CAD build for the part. Positions are in the model's coordinates, mm. A direction names the side the tool comes from. Round coordinates to 2 decimals unless told otherwise and drop trailing zeros. Loops run counter-clockwise (first coordinate to the right, second up) from the corner with the lowest first, then second, coordinate; pieces in that order, holes last.
from build123d import *

# Parameters (mm, degrees)
SKETCH1_R           = 1.75
BOSS_EXTRUDE1_DEPTH = 15
SKETCH10_R          = 1.25
CUT_EXTRUDE3_DEPTH  = 35.960692213
SKETCH11_R          = 1.95
CUT_EXTRUDE4_DEPTH  = 47.58229165
SKETCH12_R          = 3.5
BOSS_EXTRUDE8_DEPTH = 5
BOSS_EXTRUDE9_DEPTH = 15
SKETCH14_R          = 2.75
CUT_EXTRUDE5_DEPTH  = 37.697714159
FILLET1_R           = 3
FILLET2_R           = 1.5
SKETCH15_R          = 3.5
CUT_EXTRUDE6_DEPTH  = 13


with BuildPart() as part:
    # Sketch1 → Boss-Extrude1 (new body)
    with BuildSketch(Plane(origin=(0, 0, 0), x_dir=(1, 0, 0), z_dir=(0, 1, 0))):
        with BuildLine():
            Line((-4.795571708, -25.41509434), (-11.988929271, -1.037735849))
            ThreePointArc((-11.988929271, -1.037735849), (0, 15), (11.988929271, -1.037735849))
            Line((11.988929271, -1.037735849), (4.795571708, -25.41509434))
            ThreePointArc((4.795571708, -25.41509434), (0, -29), (-4.795571708, -25.41509434))
        make_face()
        with Locations(Location((0, -24, 0), (0, 0, 270))):
            Circle(SKETCH1_R, mode=Mode.SUBTRACT)
        Polygon((0, -6.437455501), (5.575, -3.218727751), (5.575, 3.218727751), (0, 6.437455501), (-5.575, 3.218727751), (-5.575, -3.218727751), align=None, mode=Mode.SUBTRACT)
    extrude(amount=BOSS_EXTRUDE1_DEPTH)

    # Sketch10 → Cut-Extrude3 (cut, through all)
    with BuildSketch(Plane(origin=(0, 0, 0), x_dir=(1, 0, 0), z_dir=(0, 1, 0))):
        with Locations(Location((0, -13, 0), (0, 0, 270))):
            Circle(SKETCH10_R)
    extrude(amount=CUT_EXTRUDE3_DEPTH, mode=Mode.SUBTRACT)

    # Sketch11 → Cut-Extrude4 (cut, through all)
    with BuildSketch(Plane(origin=(7.806004581, 0, 24.148129883), x_dir=(0.5735764363510473, 0, 0.819152044288991), z_dir=(-0.819152044288991, 0, 0.5735764363510473))):
        with Locations((-13.609353673, 7.5)):
            Circle(SKETCH11_R)
    extrude(amount=-CUT_EXTRUDE4_DEPTH, mode=Mode.SUBTRACT)

    # Sketch12 → Boss-Extrude8 (add)
    with BuildSketch(Plane(origin=(0, 0, 0), x_dir=(1, 0, 0), z_dir=(0, 1, 0))):
        Polygon((5.575, -3.218727751), (5.575, 3.218727751), (0, 6.437455501), (-5.575, 3.218727751), (-5.575, -3.218727751), (0, -6.437455501), align=None)
        with Locations(Location((0, 0, 0), (0, 0, 270))):
            Circle(SKETCH12_R, mode=Mode.SUBTRACT)
    extrude(amount=BOSS_EXTRUDE8_DEPTH)

    # Sketch13 → Boss-Extrude9 (add)
    with BuildSketch(Plane(origin=(0, 0, 0), x_dir=(1, 0, 0), z_dir=(0, 1, 0))):
        Polygon((-19.091883092, 13.435028843), (-26.162950904, 6.363961031), (-8, -11.798989873), (-8, 2.343145751), align=None)
    extrude(amount=BOSS_EXTRUDE9_DEPTH)

    # Sketch14 → Cut-Extrude5 (cut, through all)
    with BuildSketch(Plane(origin=(-9.899494937, 0, 9.899494937), x_dir=(0.707106781186549, 0, 0.707106781186546), z_dir=(-0.707106781186546, 0, 0.707106781186549))):
        with Locations((-18, 7.5)):
            Circle(SKETCH14_R)
    extrude(amount=-CUT_EXTRUDE5_DEPTH, mode=Mode.SUBTRACT)

    # Fillet1
    # the kernel refuses this fillet: 3 mm, written as the material it takes off along each edge
    with BuildSketch(Plane(origin=(-19.091883092, -7.5, -13.435028843), x_dir=(0.7071067811865492, 0, 0.7071067811865457), z_dir=(0, 1, 0))) as fillet1_piece_1:
        with BuildLine():
            CenterArc((FILLET1_R, -FILLET1_R), FILLET1_R, 90, 90)
            Line((0, -FILLET1_R), (0, 0))
            Line((0, 0), (FILLET1_R, 0))
        make_face()
    extrude(amount=30, mode=Mode.SUBTRACT)

    # Fillet2
    fillet2_edges = [part.edges().sort_by_distance(p)[0] for p in [
        (-9.153981014, 7.5, 10.645008859),
        (-11.920074413, 7.5, -6.263220163),
    ]]
    fillet(fillet2_edges, radius=FILLET2_R)

    # Sketch15 → Cut-Extrude6 (cut)
    with BuildSketch(Plane(origin=(10.275038851, 0, -7.194659659), x_dir=(0, -1, 0), z_dir=(0.819152044288991, 0, -0.5735764363510473))):
        with Locations(Location((-7.5, -10.648976576, 0), (0, 0, 90))):
            Circle(SKETCH15_R)
    extrude(amount=-CUT_EXTRUDE6_DEPTH, mode=Mode.SUBTRACT)


solid = part.part
Item 1: Cut at A-A (y = 13). List the corners of the cut face in (x, z) (3 decimals).
Verdict:
outline: (-26.163, -6.364) - (-21.213, -11.314) arc R3 ccw to (-16.971, -11.314) - (-13.507, -7.85) arc R1.5 cw to (-11.113, -8.224) arc R12.5 ccw to (11.989, 1.038) - (4.796, 25.415) arc R5 ccw to (-4.796, 25.415) - (-9.046, 11.011) arc R1.5 cw to (-9.424, 10.375) - close; hole (-5.575, -3.219) - (0, -6.437) - (5.575, -3.219) - (5.575, 3.219) - (0, 6.437) - (-5.575, 3.219) - close; hole circle Ø3.5 at (0, 24); hole circle Ø2.5 at (0, 13)
Item 2: Cut at C-C (y = 1.5). List the corners of the cut face in (x, z), plus the area to 3 significant figures.
Verdict:
outline: (-26.16, -6.36) - (-21.21, -11.31) arc R3 ccw to (-16.97, -11.31) - (-13.51, -7.85) arc R1.5 cw to (-11.11, -8.22) arc R12.5 ccw to (11.99, 1.04) - (4.8, 25.42) arc R5 ccw to (-4.8, 25.42) - (-9.05, 11.01) arc R1.5 cw to (-9.42, 10.38) - close; hole circle Ø7 at (0, 0); hole circle Ø3.5 at (0, 24); hole circle Ø2.5 at (0, 13)
area: 871 mm2
Item 3: 3-axis set-ups, long thin cutter, end or side, ignore diameter. For faces 5 (the flat face through (-2.827, 9.93, 4.806)), 6 (the flat face through (4.87, 5.99, 7.75)), 7 (the flat face through (-13.675, 5.728, -8.018)): which of +Z, -Z, +X, -X, +Y, -Y reach the whole face in a straight line?
Verdict:
face 5: +Y
face 6: none
face 7: -Z, +Y, -Y
Item 4: Cut at B-B (z = 24). List the corners of the cut face in (x, y).
Verdict:
outline: (-5.21, 0) - (-1.75, 0) - (-1.75, 15) - (-5.21, 15) - close; (1.75, 0) - (5.21, 0) - (5.21, 15) - (1.75, 15) - close
Item 5: Wall check: L1, parallel to Y at x = -20.5, z = -5; L2, parallel to X at y = 11.75, z = 13; L3, parallel to X at y = 13.5, z = -4. Give the ranges that are in metal, low to high.
Verdict:
L1: y = 0 to 4.75, 10.25 to 15
L2: x = -8.46 to -1.25, 1.25 to 8.46
L3: x = -23.8 to -4.22, 4.22 to 12.41
Item 6: Mould opens along X. For faces 1 (the cylindrical face through (-17.345, 6.447, -4.518)), 2 (the flat face through (7.643, 7.395, 15.764)), 3 (the flat face through (-23.653, 7.395, -8.873)), 4 (the flat face through (-3, 0, 7)) say: released by +X, released by -X, zero draft, split by the parting line, or undercut.
Verdict:
face 1: undercut
face 2: released by +X
face 3: released by -X
face 4: zero draft
Item 7: Flat gauge pins, fed straight in: P1, Ø7, axis at y = 10, z = -0.5, coming from the -X side; P2, Ø6, axis at x = 7, y = 12.5, coming from the +Z side; P3, Ø2, axis at y = 1.5, z = 2, coming from the -X side. Where does each tip first touch, or does it go through?
Verdict:
P1: stops at x = -23.8
P2: stops at z = 27
P3: stops at x = -18.8
Item 8: Cut at D-D (z = 19). List the corners of the cut face in (x, y).
Verdict:
outline: (-6.69, 0) - (6.69, 0) - (6.69, 15) - (-6.69, 15) - close
